Autodesk Inventor part; units mm, degrees
ref_plane "YZ Plane" through (0, 0, 0) normal (1, 0, 0) x (0, 1, 0)
ref_plane "XZ Plane" through (0, 0, 0) normal (0, 1, 0) x (-1, 0, 0)
ref_plane "XY Plane" through (0, 0, 0) normal (0, 0, 1) x (1, 0, 0)
sketch "Sketch1" plane through (0, 0, 0) normal (0, 1, 0) x (-1, 0, 0)
  line L0 (0, 0) -> (8, 0)
  line L1 (8, 0) -> (8, -20)
  line L2 (8, -20) -> (0, -20)
  line L3 (0, -20) -> (0, 0)
  line L4 (0, 0) -> (-3.7, 0)
  line L5 (-3.7, 0) -> (-3.7, -20)
  line L6 (-3.7, -20) -> (0, -20)
  line L7 (0, -20) -> (0, 0)
  line L8 (8, 0) -> (4, 0)
  line L9 (4, 0) -> (4, -5)
  line L10 (4, -5) -> (8, -5)
  line L11 (8, -5) -> (8, 0)
  line L12 (4, -5) -> (4, -15)
  circle A0 centre (4, -5) radius 2
  circle A1 centre (4, -15) radius 2
  line L13 (-7.4, 0) -> (-15.4, 0)
  line L14 (-15.4, 0) -> (-15.4, -20)
  line L15 (-15.4, -20) -> (-7.4, -20)
  line L16 (-7.4, -20) -> (-7.4, 0)
  line L17 (-7.4, 0) -> (-3.7, 0)
  line L18 (-3.7, -20) -> (-7.4, -20)
  line L19 (-7.4, -20) -> (-7.4, 0)
  line L20 (-15.4, 0) -> (-11.4, 0)
  line L21 (-11.4, 0) -> (-11.4, -5)
  line L22 (-11.4, -5) -> (-15.4, -5)
  line L23 (-15.4, -5) -> (-15.4, 0)
  line L24 (-11.4, -5) -> (-11.4, -15)
  circle A2 centre (-11.4, -5) radius 2
  circle A3 centre (-11.4, -15) radius 2
  dimension "d0" = 8
  dimension "d1" = 20
  dimension "d2" = 3.7
  dimension "d3" = 4
  dimension "d4" = 5
  dimension "d5" = 10
  dimension "d6" = 4
  dimension "d7" = 4
extrude "Extrusion1" add sketch "Sketch1" along normal blind 4 contours L0 L9 A0 L10 L1 L2 L3 | L3 L6 L5 L4 | L0 L1 L10 A0 L9 | L5 L18 L16 L17 | L16 L15 L14 L22 A2 L21 L13 | L21 A2 L22 L14 L13
fillet "Fillet1" radius 4 4 edges at (-8, 2, 0) (15.4, 2, 0) (15.4, 2, -20) (-8, 2, -20)
sketch "Sketch2" plane through (0, 4, 0) normal (0, 1, 0) x (1, 0, 0)
  line L0 (-8, 16) -> (-8, 4)
  line L1 (-8, 10) -> (15.4, 10)
  line L2 (15.4, 4) -> (15.4, 16)
  line L3 (11.4, 20) -> (-4, 20)
  line L4 (1.2, 0) -> (6.2, 0)
  line L5 (6.2, 0) -> (6.2, 20)
  line L6 (6.2, 20) -> (1.2, 20)
  line L7 (1.2, 20) -> (1.2, 0)
  line L8 (1.2, 0) -> (6.2, 20) construction
  line L9 (6.2, 0) -> (1.2, 20) construction
  point P0 (0, 0)
  point P1 (3.7, 10)
  point P2 (1.2, 20)
  dimension "d11" = 5
extrude "Extrusion2" add sketch "Sketch2" along normal blind 30
sketch "Sketch3" plane through (0, 34, 0) normal (0, 1, 0) x (1, 0, 0)
  line L0 (6.2, 20) -> (6.2, 0)
  line L1 (1.2, 0) -> (1.2, 20)
  line L2 (6.2, 0) -> (1.2, 0)
  line L3 (1.2, 0) -> (1.2, 6)
  line L4 (1.2, 6) -> (6.2, 6)
  line L5 (6.2, 6) -> (6.2, 0)
  line L6 (1.2, 6) -> (-8, 6)
  line L7 (-8, 6) -> (-8, 0)
  line L8 (-8, 0) -> (1.2, 0)
  line L9 (1.2, 0) -> (1.2, 6)
  line L10 (6.2, 6) -> (15.4, 6)
  line L11 (15.4, 6) -> (15.4, 0)
  line L12 (15.4, 0) -> (6.2, 0)
  line L13 (6.2, 0) -> (6.2, 6)
  line L14 (-8, 0) -> (-5, 0)
  line L15 (-5, 0) -> (-5, 3)
  line L16 (-5, 3) -> (-8, 3)
  line L17 (-8, 3) -> (-8, 0)
  line L18 (15.4, 0) -> (12.4, 0)
  line L19 (12.4, 0) -> (12.4, 3)
  line L20 (12.4, 3) -> (15.4, 3)
  line L21 (15.4, 3) -> (15.4, 0)
  circle A0 centre (-5, 3) radius 1.5
  circle A1 centre (12.4, 3) radius 1.5
  point P0 (0, 0)
  dimension "d14" = 6
  dimension "d15" = 6
  dimension "d16" = 6
  dimension "d17" = 3
  dimension "d18" = 3
  dimension "d19" = 3
  dimension "d20" = 3
  dimension "d21" = 3
  dimension "d22" = 3
extrude "Extrusion3" add sketch "Sketch3" against normal blind 5 contours L10 L11 L20 A1 L19 L12 L0 | L1 L8 L15 A0 L16 L7 L6 | L19 A1 L20 L11 L12 | L8 L7 L16 A0 L15
fillet "Fillet2" radius 2 4 edges at (1.2, 31.5, -6) (6.2, 31.5, -6) (6.2, 29, -3) (1.2, 29, -3)
chamfer "Chamfer1" distance 12 distance2 30 1 edges at (3.7, 34, -20) measured on face at (2.8667, 34, -16)
properties part number "rigid_support3"
Geometry: final body of the model. Coordinates: model frame, mm. A direction names the side the tool comes from. Give positions to 0.01 mm unless a question says otherwise; leave off trailing zeros. Write each loop counter-clockwise with the first axis right and the second up, starting at its lowest first coordinate (ties: lowest second). Pieces come first, ordered by that corner, then holes. Notation, with made-up numbers: M -18.5,84.5 L -5.5,84.5 A11 ccw -5.5,89.5 Z; hole C -4.5,63.5 d1. An arc over 180 degrees is marked long. Answer in a Markdown table with one row per item. Add a question column.
(1) Section C-C on x = -5.5. Return loops of the section in (y, z).
(2) Reachability of faces 1 (the cylindrical face through (-2.526, 1.972, -6.352)), 2 (the cylindrical face through (0.6, 28.43, -3.17)), 3 (the cylindrical face through (-6.2, 31.5, -2.1)), 4 (the cylindrical face through (6.8, 28.43, -3.06)), 5 (the flat face through (12, 32, -6)) from +Z, -Z, +X, -X, +Y, -Y: full face, straight path, thin tool, end or side. Return the list, or none.
(3) Section A-A on z = -5. Return loops of the section in (x, y).
(4) Mould query, pull axis Z, two halves, no side actions, for faces 6 (the cylindrical face through (6.8, 31.23, -6.57)), 7 (the cylindrical face through (14.197, 2.028, -1.141)), 8 (the cylindrical face through (-4, 2, -17)), 9 (the flat face through (11, 4, -10)). Classes: +Z half, -Z half, draft (parallel to the pull), parting line (faces both ways), or undercut.
(5) Ray query, line 1 (X direction, y = 31.2, z = -3); line 2 (Z direction, x = 11.4, y = 2.1); line 3 (X direction, y = 2, z = -6.5). Return the intervals inside material, ascending.
(6) Section D-D on y = 32. Return loops of the section in (x, z).
(7) Section B-B on y = 3. Return loops of the section in (x, z), and give its area (3 significant figures).
(8) First-contact query: pin 1 (5.5 mm diameter, centred on x = 10.5, y = 31, fed in from -Z); pin 2 (2.5 mm diameter, centred on x = -3.5, y = 30.5, fed in from -Z); pin 3 (2.5 mm diameter, centred on x = -5, z = -3, fed in from +Y). Flat tips, straight axial feed; report the tip coordinate or a pass-through.
Result set:
| question | item | result |
|---|---|---|
| 1 | outline | M 0,-19.71 L 4,-19.71 L 4,-16.32 L 0,-16.32 Z; M 0,-13.68 L 4,-13.68 L 4,-6.32 L 0,-6.32 Z; M 0,-3.68 L 4,-3.68 L 4,-0.29 L 0,-0.29 Z; M 29,-6 L 34,-6 L 34,-4.41 L 29,-4.41 Z; M 29,-1.59 L 34,-1.59 L 34,0 L 29,0 Z |
| 2 | face 1 | -Y |
| 2 | face 2 | +Z, -Z, -X |
| 2 | face 3 | +Y |
| 2 | face 4 | +Z, -Z, +X |
| 2 | face 5 | -Z, +X, +Y |
| 3 | outline | M -8,0 L -6,0 L -6,4 L -8,4 Z; M -8,29 L -0.8,29 A2 cw 1.2,27 L 1.2,4 L -2,4 L -2,0 L 9.4,0 L 9.4,4 L 6.2,4 L 6.2,27 A2 cw 8.2,29 L 15.4,29 L 15.4,34 L -8,34 Z; M 13.4,0 L 15.4,0 L 15.4,4 L 13.4,4 Z |
| 4 | face 6 | -Z half |
| 4 | face 7 | +Z half |
| 4 | face 8 | undercut |
| 4 | face 9 | draft |
| 5 | line 1 | x = -8 to -6.5, -3.5 to 10.9, 13.9 to 15.4 |
| 5 | line 2 | z = -20 to -17, -13 to -7, -3 to 0 |
| 5 | line 3 | x = -8 to -5.32, -2.68 to 10.08, 12.72 to 15.4 |
| 6 | outline | M -8,-6 L -0.8,-6 A2 cw 1.2,-8 L 1.2,-8.8 L 6.2,-8.8 L 6.2,-8 A2 cw 8.2,-6 L 15.4,-6 L 15.4,0 L -8,0 Z; hole C -5,-3 d3; hole C 12.4,-3 d3 |
| 7 | outline | M -8,-16 A4 ccw -4,-20 L 11.4,-20 A4 ccw 15.4,-16 L 15.4,-4 A4 ccw 11.4,0 L -4,0 A4 ccw -8,-4 Z; hole C -4,-15 d4; hole C -4,-5 d4; hole C 11.4,-15 d4; hole C 11.4,-5 d4 |
| 7 | area | 404 mm^2 |
| 8 | pin 1 | stops at z = -6.05 |
| 8 | pin 2 | stops at z = -6 |
| 8 | pin 3 | stops at y = 4 |
